Part print with two shaded views. Sizes in mm from the minimum x, y, z corner. A direction names the side the tool comes from. Coordinates: 2 decimals unless noted, no trailing zeros. Loops run counter-clockwise (first coordinate to the right, second up) from the corner with the lowest first, then second, coordinate; pieces in that order, holes last. Notation, with made-up numbers: (65.5, -10.5) -> (86.5, -10.5) arc R19 cw to (86.5, 14.5) -> close; hole circle Ø6 at (74, -19.5). An arc over 180 degrees is marked (long way). One line per item, written item: value. Start each with the question number.
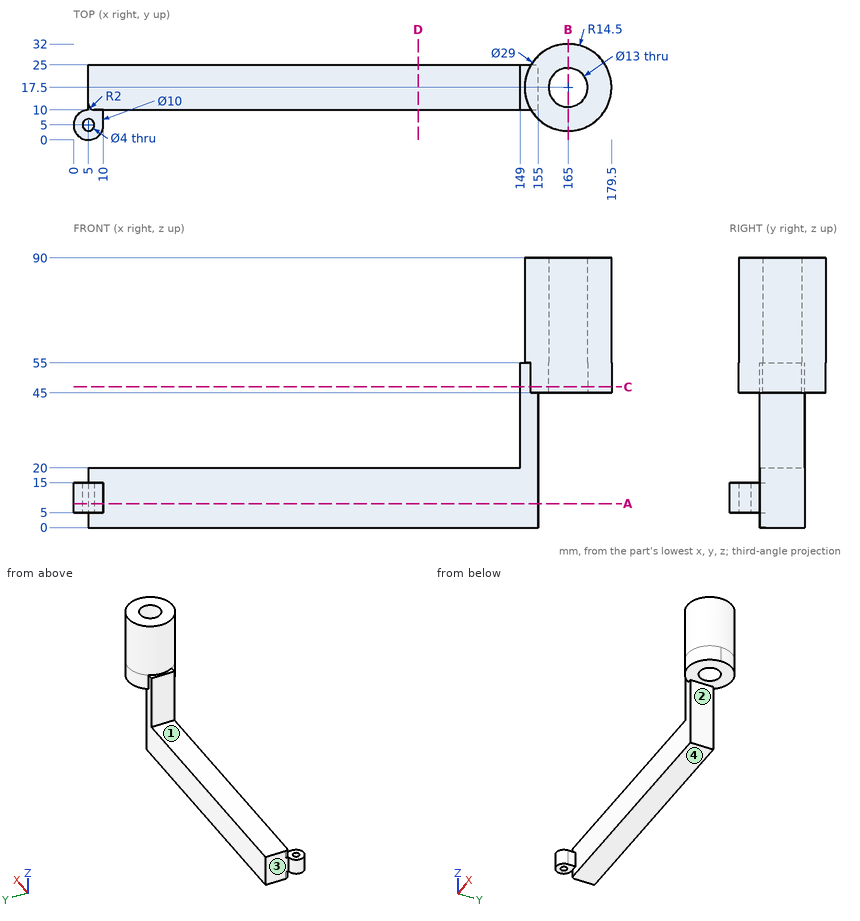
Item 1: Band-saw the part on B-B, the plane x = 165. List the corners of the cut face in (y, z).
Item 2: Band-saw the part on A-A, the plane z = 8. List the corners of the cut face in (x, y).
Item 3: Probe probe 1 along Y at (x, z) = (165, 72); probe 2 along X at (y, z) = (17, 51); probe 3 along Z at (x, y) = (94.5, 17.5). List the from-to ranges inside material, lowest first.
Item 4: Tool access for the marked faces 1, 2, 3 and 4: list every direction of +Z, -Z, +X, -X, +Y, -Y with a clear straight run to the whole face (end or side of a thin tool).
Item 5: Drop flat-ended pins along their axis: pin 1 Ø1.5 at (y, z) = (8.5, 9.5) entering from +X; pin 2 Ø6.5 at (x, y) = (5, 5) entering from +Z; pin 3 Ø8 at (y, z) = (26, 34) entering from +X. Give the stop position or say it passes through.
Item 6: Band-saw the part on D-D, the plane x = 115. List the corners of the cut face in (y, z).
Item 7: Band-saw the part on C-C, the plane z = 47. List the corners of the cut face in (x, y).
Worked out:
1. outline: (3, 45) -> (11, 45) -> (11, 90) -> (3, 90) -> close; (24, 45) -> (32, 45) -> (32, 90) -> (24, 90) -> close
2. outline: (5, 10) arc R5 ccw (long way) to (10, 5) -> (10, 10) -> (155, 10) -> (155, 25) -> (5, 25) -> close; hole circle Ø4 at (5, 5)
3. probe 1: y = 3 to 11, 24 to 32
3. probe 2: x = 149 to 158.52, 171.48 to 179.49
3. probe 3: z = 0 to 20
4. face 1: +Z, -X, +Y, -Y
4. face 2: -Z, +X, +Y, -Y
4. face 3: +Z, -Z, -X, +Y
4. face 4: -Z, +X, -X, +Y, -Y
5. pin 1: stops at x = 10
5. pin 2: stops at z = 15
5. pin 3: stops at x = 155
6. outline: (10, 0) -> (25, 0) -> (25, 20) -> (10, 20) -> close
7. outline: (149, 10) -> (152.59, 10) arc R14.5 ccw (long way) to (152.59, 25) -> (149, 25) -> close; hole circle Ø13 at (165, 17.5)
